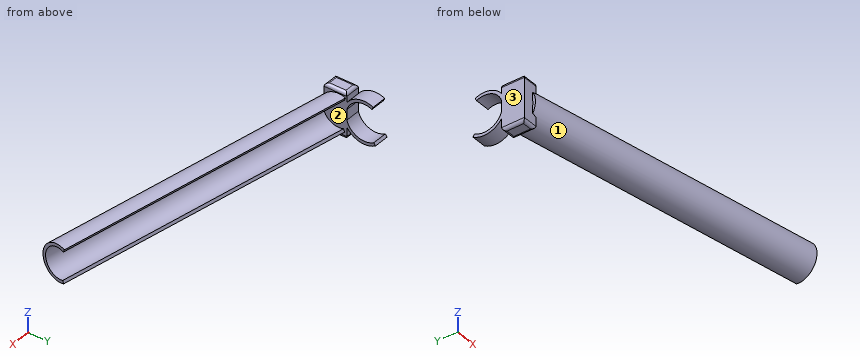
```python
from build123d import *

# Parameters (mm, degrees)
EXTRUDE_1_DEPTH      = 10
SKETCH_2_W           = 10
SKETCH_2_H           = 30
EXTRUDE_1_2_DEPTH    = 2.5
EXTRUDE_4_DEPTH      = 200
EXTRUDE_4_DEPTH_BACK = 1
SKETCH_8_W           = 10
SKETCH_8_H           = 30
EXTRUDE_2_DEPTH      = 10
FILLET_2_R           = 2


with BuildPart() as part:
    # Sketch 1 → Extrude 1 (new body)
    with BuildSketch(Plane(origin=(0, 0, 0), x_dir=(0, 0, -1), z_dir=(1, 0, 0))):
        with BuildLine():
            ThreePointArc((-10.846142842, 5.134314505), (0.719237504, -11.978426333), (10.153857158, 6.39524705))
            Line((10.153857158, 6.39524705), (11.846166684, 7.461121558))
            ThreePointArc((11.846166684, 7.461121558), (0.839110422, -13.974830722), (-12.653833316, 5.99003359))
            Line((-12.653833316, 5.99003359), (-10.846142842, 5.134314505))
        make_face()
    extrude(amount=EXTRUDE_1_DEPTH)

    # Sketch 2 → Extrude 1 2 (add, symmetric)
    with BuildSketch(Plane(origin=(0, -14, 0), x_dir=(-1, 0, 0), z_dir=(0, -1, 0))):
        with Locations((-5, 1)):
            Rectangle(SKETCH_2_W, SKETCH_2_H)
    extrude(amount=EXTRUDE_1_2_DEPTH, both=True)



with BuildPart() as body_2:
    # Sketch 6 → Extrude 4 (new, two sides: drawn at the far end of the back side and taken through both)
    with BuildSketch(Plane(origin=(12.520129286, -2.207636595, 0), x_dir=(0, 0, 1), z_dir=(0.984807753012208, -0.17364817766693072, 0)).offset(-EXTRUDE_4_DEPTH_BACK)):
        with BuildLine():
            ThreePointArc((-11.782684324, 11.014511571), (-0.139277573, 26.995609574), (10.62288968, 10.40825987))
            Line((10.62288968, 10.40825987), (8.775098788, 11.173549892))
            ThreePointArc((8.775098788, 11.173549892), (-0.193373923, 24.996341312), (-9.896212883, 11.678759642))
            Line((-9.896212883, 11.678759642), (-11.782684324, 11.014511571))
        make_face()
    extrude(amount=EXTRUDE_4_DEPTH + EXTRUDE_4_DEPTH_BACK)


with BuildPart() as part_1:
    add(part.part)

    add(body_2.part)  # Extrude 2 merges body 2
    # Sketch 8 → Extrude 2 (add)
    with BuildSketch(Plane.XZ.offset(16.5)):
        with Locations((5, -1)):
            Rectangle(SKETCH_8_W, SKETCH_8_H)
    extrude(amount=EXTRUDE_2_DEPTH)

    # Fillet 2
    fillet_2_edges = [part_1.edges().sort_by_distance(p)[0] for p in [
        (10, -19, -16),
        (5, -11.5, 14),
        (10, -19, 14),
        (0, -19, 14),
        (5, -11.5, -16),
        (0, -19, -16),
        (5, -26.5, -16),
        (5, -26.5, 14),
    ]]
    fillet(fillet_2_edges, radius=FILLET_2_R)


solid = part_1.part
```
The listing builds one solid part. Answer for the finished solid, in the listing's coordinates (mm). Face numbers are marked on the shaded views. Coordinates: 2 decimals unless noted, no trailing zeros. Order: outer loops, then holes, each group sorted by start corner. A loop starts at its lowest first (then second) coordinate and runs counter-clockwise, first axis right, second up. Notation, with made-up numbers: M 15,78 L 23,78 A10 ccw 23,82 Z; hole C 79.5,-14 d6. An arc over 180 degrees is marked long. Answer as a JSON object with one key per item and string values. Group by question number.
1. Flat-ended cylindrical pins translate along their axes: P1, Ø6, axis at x = 57, y = -23.5, coming from the -Z side; P2, Ø14, axis at y = -4, z = 4, coming from the +X side; P3, Ø8, axis at y = 0.5, z = -11, coming from the -X side; P4, Ø3.5, axis at x = 2.5, z = -1, coming from the +Y side. Find the tip coordinate at first contact, or state that the pin passes through.
2. Determine the mould class of the marked faces 1, 2 and 3 for opening direction Z: released by +Z, released by -Z, zero draft, split by the parting line, or undercut.
3. Straight lines are drawn through the part: line 1 (Z direction, x = 185.5, y = -47); line 2 (X direction, y = -18, z = -13.5); line 3 (Z direction, x = 118, y = -43). For each, find the intervals that lie inside material, in ascending order.
4. Section A-A on y = -9 is taken. Write down the section's boundary in (x, z).
Values follow:
{
 "1": {"P1": "z = -12.46", "P2": "x = 10", "P3": "x = 0", "P4": "y = -11.5"},
 "2": {"face 1": "split by the parting line", "face 2": "undercut", "face 3": "zero draft"},
 "3": {"line 1": "-12.43 to -10.42, 9.49 to 11.5", "line 2": "0 to 10", "line 3": "-10.31 to -7.74, 6.82 to 9.38"},
 "4": {"outline": "M 0,-10.72 L 10,-10.72 L 10,-7.94 L 0,-7.94 Z; M 0,7.94 L 10,7.94 L 10,10.72 L 0,10.72 Z"}
}
